Geometry check sheet. Reference: the model listing, model coordinates, mm. A direction names the side the tool comes from. Give positions to 0.01 mm unless a question says otherwise; leave off trailing zeros. Loops run counter-clockwise (first coordinate to the right, second up) from the corner with the lowest first, then second, coordinate; pieces in that order, holes last. Notation, with made-up numbers: (75, 36.25) -> (107, 36.25) arc R26 ccw to (107, 70.25) -> close; hole circle Ø7 at (-1.5, 29). An arc over 180 degrees is marked (long way). Answer in a Markdown table with one row per item. Add a question column.
```python
from build123d import *

# Parameters (mm, degrees)
SKETCH1_R             = 33.75
BOSS_EXTRUDE1_DEPTH   = 5
SKETCH2_R             = 33.6
BOSS_EXTRUDE2_DEPTH   = 0.1
SKETCH3_R             = 33.75
BOSS_EXTRUDE3_DEPTH   = 79.3
SKETCH4_R             = 33.6
BOSS_EXTRUDE4_DEPTH   = 0.1
SKETCH5_R             = 33.75
BOSS_EXTRUDE5_DEPTH   = 5
SKETCH6_R             = 5
CUT_EXTRUDE1_DEPTH    = 5
SKETCH7_R             = 4.9
SKETCH7_R_2           = 4.4
BOSS_EXTRUDE6_DEPTH   = 5
SKETCH8_R             = 4
BOSS_EXTRUDE7_DEPTH   = 24.5
SKETCH9_R             = 15
BOSS_EXTRUDE8_DEPTH   = 9.91
M5_TAPPED_HOLE1_D     = 4.2
M5_TAPPED_HOLE1_DEPTH = 5
M5_TAPPED_HOLE1_TIP   = 1.2618073
SKETCH12_W            = 8
SKETCH12_H            = 10
CUT_EXTRUDE2_DEPTH    = 1
SKETCH13_R            = 4
BOSS_EXTRUDE9_DEPTH   = 1
SKETCH14_R            = 3.8
BOSS_EXTRUDE10_DEPTH  = 1
SKETCH15_R            = 4
BOSS_EXTRUDE11_DEPTH  = 3
SKETCH16_R            = 3
CUT_EXTRUDE3_DEPTH    = 3


with BuildPart() as part:
    # Sketch1 → Boss-Extrude1 (new body)
    with BuildSketch(Plane.XY):
        Circle(SKETCH1_R)
    extrude(amount=BOSS_EXTRUDE1_DEPTH)

    # Sketch2 → Boss-Extrude2 (add)
    with BuildSketch(Plane.XY.offset(5)):
        Circle(SKETCH2_R)
    extrude(amount=BOSS_EXTRUDE2_DEPTH)

    # Sketch3 → Boss-Extrude3 (add)
    with BuildSketch(Plane.XY.offset(5.1)):
        Circle(SKETCH3_R)
    extrude(amount=BOSS_EXTRUDE3_DEPTH)

    # Sketch4 → Boss-Extrude4 (add)
    with BuildSketch(Plane.XY.offset(84.4)):
        Circle(SKETCH4_R)
    extrude(amount=BOSS_EXTRUDE4_DEPTH)

    # Sketch5 → Boss-Extrude5 (add)
    with BuildSketch(Plane.XY.offset(84.5)):
        Circle(SKETCH5_R)
    extrude(amount=BOSS_EXTRUDE5_DEPTH)

    # Sketch6 → Cut-Extrude1 (cut)
    with BuildSketch(Plane.XY.offset(89.5)):
        Circle(SKETCH6_R)
    extrude(amount=-CUT_EXTRUDE1_DEPTH, mode=Mode.SUBTRACT)

    # Sketch7 → Boss-Extrude6 (add)
    with BuildSketch(Plane.XY.offset(84.5)):
        Circle(SKETCH7_R)
        Circle(SKETCH7_R_2, mode=Mode.SUBTRACT)
    extrude(amount=BOSS_EXTRUDE6_DEPTH)

    # Sketch8 → Boss-Extrude7 (add)
    with BuildSketch(Plane.XY.offset(84.5)):
        Circle(SKETCH8_R)
    extrude(amount=BOSS_EXTRUDE7_DEPTH)

    # Sketch9 → Boss-Extrude8 (add)
    with BuildSketch(Plane(origin=(0, 0, 0), x_dir=(-1, 0, 0), z_dir=(0, 0, -1))):
        Circle(SKETCH9_R)
    extrude(amount=BOSS_EXTRUDE8_DEPTH)

    # M5 Tapped Hole1
    with Locations(Plane(origin=(-20.308390576, 5.345023126, 89.5), x_dir=(1, 0, 0), z_dir=(0, 0, 1))):
        with Locations((0, 0), (35.091511675, 9.57004746), (25.833660053, -25.605116838)):
            Hole(M5_TAPPED_HOLE1_D / 2, depth=M5_TAPPED_HOLE1_DEPTH)
            with Locations((0, 0, -(M5_TAPPED_HOLE1_DEPTH + M5_TAPPED_HOLE1_TIP / 2))):  # 118° drill point
                Cone(0, M5_TAPPED_HOLE1_D / 2, M5_TAPPED_HOLE1_TIP, mode=Mode.SUBTRACT)

    # Sketch12 → Cut-Extrude2 (cut)
    with BuildSketch(Plane(origin=(0, 4, 0), x_dir=(1, 0, 0), z_dir=(0, 1, 0))):
        with Locations((0, -104)):
            Rectangle(SKETCH12_W, SKETCH12_H)
    extrude(amount=-CUT_EXTRUDE2_DEPTH, mode=Mode.SUBTRACT)

    # Sketch13 → Boss-Extrude9 (add)
    with BuildSketch(Plane.XY.offset(109)):
        Circle(SKETCH13_R)
    extrude(amount=BOSS_EXTRUDE9_DEPTH)

    # Sketch14 → Boss-Extrude10 (add)
    with BuildSketch(Plane.XY.offset(110)):
        Circle(SKETCH14_R)
    extrude(amount=BOSS_EXTRUDE10_DEPTH)

    # Sketch15 → Boss-Extrude11 (add)
    with BuildSketch(Plane.XY.offset(111)):
        Circle(SKETCH15_R)
    extrude(amount=BOSS_EXTRUDE11_DEPTH)

    # Sketch16 → Cut-Extrude3 (cut)
    with BuildSketch(Plane.XY.offset(89.5)):
        with Locations((0, 28)):
            Circle(SKETCH16_R)
        with Locations((0, -28)):
            Circle(SKETCH16_R)
    extrude(amount=-CUT_EXTRUDE3_DEPTH, mode=Mode.SUBTRACT)


solid = part.part
```
1. Sectioned sample at D-D (x = -25). Enter the section's corners in (y, z).
2. Material ranges on L1, parallel to Z at x = 1.5, y = -6.5; L2, parallel to Y at x = 4.5, z = 86; L3, parallel to Z at x = 29, y = 15, recorded low to high. Write a range as from..to.
3. Gauge pin test, flat ends, axial feed: pin 1 Ø1.5 at (x, z) = (-24, 84) entering from -Y; pin 2 Ø5 at (x, z) = (24.5, 16) entering from +Y; pin 3 Ø6.5 at (x, y) = (14.78, 14.92) entering from +Z. Record the tip position at first contact, or that the pin passes through.
4. Sectioned sample at B-B (z = 38.5). Enter the section's corners in (x, y), plus the area to 3 significant figures.
5. Access from +Z, -Z, +X, -X, +Y, -Y to the whole of each face (thin tool, end or side, straight path). Record for faces 1 (the face through (-26.78, -20.54, 86.96)), 2 (the face through (-0.867, -3.905, 112.479)).
6. Sectioned sample at A-A (x = -10.5). Enter the section's corners in (y, z), plus the area to 3 significant figures.
7. Sectioned sample at C-C (y = -28). Enter the section's corners in (x, z).
Response:
| question | item | result |
|---|---|---|
| 1 | outline | (-22.67, 0) -> (22.67, 0) -> (22.67, 5) -> (22.45, 5) -> (22.45, 5.1) -> (22.67, 5.1) -> (22.67, 84.4) -> (22.45, 84.4) -> (22.45, 84.5) -> (22.67, 84.5) -> (22.67, 89.5) -> (-22.67, 89.5) -> (-22.67, 84.5) -> (-22.45, 84.5) -> (-22.45, 84.4) -> (-22.67, 84.4) -> (-22.67, 5.1) -> (-22.45, 5.1) -> (-22.45, 5) -> (-22.67, 5) -> close |
| 2 | L1 | z = -9.91..89.5 |
| 2 | L2 | y = -33.45..-22.09, -18.43..-2.18, -1.94..1.94, 2.18..33.45 |
| 2 | L3 | z = 0..89.5 |
| 3 | pin 1 | stops at y = -24.46 |
| 3 | pin 2 | stops at y = 25.59 |
| 3 | pin 3 | stops at z = 89.5 |
| 4 | outline | circle Ø67.5 at (0, 0) |
| 4 | area | 3,580 mm2 |
| 5 | face 1 | +Z, -Z |
| 5 | face 2 | +Z |
| 6 | outline | (-32.08, 0) -> (-10.71, 0) -> (-10.71, -9.91) -> (10.71, -9.91) -> (10.71, 0) -> (32.08, 0) -> (32.08, 5) -> (31.92, 5) -> (31.92, 5.1) -> (32.08, 5.1) -> (32.08, 84.4) -> (31.92, 84.4) -> (31.92, 84.5) -> (32.08, 84.5) -> (32.08, 89.5) -> (-32.08, 89.5) -> (-32.08, 84.5) -> (-31.92, 84.5) -> (-31.92, 84.4) -> (-32.08, 84.4) -> (-32.08, 5.1) -> (-31.92, 5.1) -> (-31.92, 5) -> (-32.08, 5) -> close |
| 6 | area | 5,950 mm2 |
| 7 | outline | (-18.84, 0) -> (18.84, 0) -> (18.84, 5) -> (18.57, 5) -> (18.57, 5.1) -> (18.84, 5.1) -> (18.84, 84.4) -> (18.57, 84.4) -> (18.57, 84.5) -> (18.84, 84.5) -> (18.84, 89.5) -> (3, 89.5) -> (3, 86.5) -> (-3, 86.5) -> (-3, 89.5) -> (-18.84, 89.5) -> (-18.84, 84.5) -> (-18.57, 84.5) -> (-18.57, 84.4) -> (-18.84, 84.4) -> (-18.84, 5.1) -> (-18.57, 5.1) -> (-18.57, 5) -> (-18.84, 5) -> close |
